```python
from build123d import *

# Parameters (mm, degrees)
F0_W      = 107.95
F0_H      = 63.5
F1_DEPTH  = 57.15
F2_W      = 44.45
F2_H      = 31.75
F3_DEPTH  = 31.75
F4_W      = 63.5
F4_H      = 31.75
F5_DEPTH  = 44.45
F6_W      = 6.35
F6_H      = 6.35
F7_DEPTH  = 57.151
F9_DEPTH  = 31.75
F10_W     = 12.7
F10_H     = 63.5
F11_DEPTH = 25.4
F13_DEPTH = 25.401
F14_R     = 6.35
F15_DEPTH = 25.401
F17_DEPTH = 63.501


with BuildPart() as f1:
    # F0 (on Front) → F1 (new body)
    with BuildSketch(Plane.XZ):
        with Locations((53.975, 31.75)):
            Rectangle(F0_W, F0_H)
    extrude(amount=-F1_DEPTH)

    # F2 (on face) → F3 (cut)
    with BuildSketch(Plane.XY.offset(63.5)):
        with Locations((22.225, 15.875)):
            Rectangle(F2_W, F2_H)
    extrude(amount=-F3_DEPTH, mode=Mode.SUBTRACT)

    # F4 (on face) → F5 (cut)
    with BuildSketch(Plane.XY.offset(63.5)):
        with Locations((76.2, 15.875)):
            Rectangle(F4_W, F4_H)
    extrude(amount=-F5_DEPTH, mode=Mode.SUBTRACT)

    # F6 (on Front) → F7 (cut, through all)
    with BuildSketch(Plane.XZ):
        with Locations((3.175, 3.175)):
            Rectangle(F6_W, F6_H)
    extrude(amount=-F7_DEPTH, mode=Mode.SUBTRACT)

    # F8 (on face) → F9 (cut)
    with BuildSketch(Plane.XZ):
        Polygon((44.45, 12.7), (44.45, 0), (107.95, 0), (107.95, 19.05), (57.15, 19.05), (57.15, 12.7), align=None)
    extrude(amount=-F9_DEPTH, mode=Mode.SUBTRACT)

    # F10 (on face) → F11 (cut)
    with BuildSketch(Plane.XZ.offset(-31.75)):
        with Locations((101.6, 31.75)):
            Rectangle(F10_W, F10_H)
    extrude(amount=-F11_DEPTH, mode=Mode.SUBTRACT)

    # F12 (on face) → F13 (cut, through all)
    with BuildSketch(Plane.XZ.offset(-31.75)):
        Polygon((95.25, 63.5), (50.8, 63.5), (95.25, 19.05), align=None)
    extrude(amount=-F13_DEPTH, mode=Mode.SUBTRACT)

    # F14 (on face) → F15 (cut, through all)
    with BuildSketch(Plane.XZ.offset(-31.75)):
        with Locations((19.05, 50.8)):
            Circle(F14_R)
    extrude(amount=-F15_DEPTH, mode=Mode.SUBTRACT)

    # F16 (on Top) → F17 (cut, through all)
    with BuildSketch(Plane.XY):
        Polygon((95.25, 38.1), (95.25, 57.15), (76.2, 57.15), align=None)
    extrude(amount=F17_DEPTH, mode=Mode.SUBTRACT)


solid = f1.part
```
Input: part model. Units: mm. Frame: model coordinates. A direction names the side the tool comes from. Give positions to 0.01 mm unless a question says otherwise; leave off trailing zeros. Write each loop counter-clockwise with the first axis right and the second up, starting at its lowest first coordinate (ties: lowest second). Pieces come first, ordered by that corner, then holes. Notation, with made-up numbers: (43.5, 47.5) - (86.5, 47.5) arc R16 cw to (86.5, 71.5) - close; hole circle Ø1 at (53, 51). An arc over 180 degrees is marked (long way). Write item = value, one per line. Start each with the question number.
1. Ray query, L1, parallel to Z at x = 19, y = 38; L2, parallel to X at y = 10, z = 3; L3, parallel to Y at x = 40, z = 35. Return the intervals inside material, ascending.
2. Access query for faces 1 (the flat face through (57.15, 16, 16)), 2 (the flat face through (51, 16, 12.7)), 3 (the flat face through (3, 28, 6.35)), 4 (the flat face through (44.45, 16, 25)), 5 (the flat face through (22, 16, 31.75)). Directions: +Z, -Z, +X, -X, +Y, -Y. A direction counts if a zero-diameter tool reaches every point of the face in a straight line with its end or side. Return the directions, or none.
3. Section query B-B, the plane x = 19.05. Output: boundary loops of the cut face in (y, z).
4. First-contact query: pin 1 Ø10 at (y, z) = (20.5, 7.5) entering from +X; pin 2 Ø14 at (x, y) = (49.5, 21) entering from +Z; pin 3 Ø1.9 at (y, z) = (34, 4) entering from -X. Flat tips, straight axial feed; report the tip coordinate or a pass-through.
5. Section query A-A, the plane z = 50.8. Output: boundary loops of the cut face in (x, y), then the cut area to 3 significant figures.
6. Section query C-C, the plane y = 42.5. Output: boundary loops of the cut face in (x, z), then the cut area to 3 significant figures.
7. Section query D-D, the plane y = 15.5. Output: boundary loops of the cut face in (x, z).
8. Mould query, pull axis X, two halves, no side actions, for faces 6 (the flat face through (6.35, 28, 3)), 7 (the flat face through (44.45, 16, 6)), 8 (the flat face through (40, 35, 0)), 9 (the cylindrical face through (22.464, 44.272, 56.154)). Classes: released by +X, released by -X, zero draft, split by the parting line, or undercut.
Check sheet entries:
q1.L1 = 0 to 44.45, 57.15 to 63.5
q1.L2 = 6.35 to 44.45
q1.L3 = 31.75 to 57.15
q2.face_1 = +Z, -Z, +X, -Y
q2.face_2 = -Z, +X, -Y
q2.face_3 = -Z, -X, +Y, -Y
q2.face_4 = +Z, +X, -Y
q2.face_5 = +Z, +X, -X, -Y
q3.outline = (0, 0) - (57.15, 0) - (57.15, 44.45) - (31.75, 44.45) - (31.75, 31.75) - (0, 31.75) - close; (31.75, 57.15) - (57.15, 57.15) - (57.15, 63.5) - (31.75, 63.5) - close
q4.pin_1 = 44.45
q4.pin_2 = 31.75
q4.pin_3 = 6.35
q5.outline = (0, 31.75) - (12.7, 31.75) - (12.7, 57.15) - (0, 57.15) - close; (25.4, 31.75) - (63.5, 31.75) - (63.5, 57.15) - (25.4, 57.15) - close
q5.area = 1,290 mm2
q6.outline = (0, 6.35) - (6.35, 6.35) - (6.35, 0) - (90.85, 0) - (90.85, 23.45) - (50.8, 63.5) - (0, 63.5) - close; hole circle Ø12.7 at (19.05, 50.8)
q6.area = 4,800 mm2
q7.outline = (0, 6.35) - (6.35, 6.35) - (6.35, 0) - (44.45, 0) - (44.45, 12.7) - (57.15, 12.7) - (57.15, 19.05) - (44.45, 19.05) - (44.45, 31.75) - (0, 31.75) - close
q8.face_6 = released by -X
q8.face_7 = released by +X
q8.face_8 = zero draft
q8.face_9 = undercut
